```python
from build123d import *

# Parameters (mm, degrees)
SKETCH1_W           = 70
SKETCH1_H           = 75
BOSS_EXTRUDE1_DEPTH = 9
SKETCH2_W           = 65.1
SKETCH2_H           = 70.1
CUT_EXTRUDE1_DEPTH  = 4
SKETCH4_R           = 2.5
BOSS_EXTRUDE3_DEPTH = 7.5
FILLET1_R           = 0.4


with BuildPart() as part:
    # Sketch1 → Boss-Extrude1 (new body)
    with BuildSketch(Plane(origin=(0, 0, 0), x_dir=(1, 0, 0), z_dir=(0, 1, 0))):
        with Locations((35, 37.5)):
            Rectangle(SKETCH1_W, SKETCH1_H)
    extrude(amount=BOSS_EXTRUDE1_DEPTH)

    # Sketch2 → Cut-Extrude1 (cut)
    with BuildSketch(Plane(origin=(0, 9, 0), x_dir=(1, 0, 0), z_dir=(0, 1, 0))):
        with Locations((35, 37.5)):
            Rectangle(SKETCH2_W, SKETCH2_H)
    extrude(amount=-CUT_EXTRUDE1_DEPTH, mode=Mode.SUBTRACT)

    # Sketch4 → Boss-Extrude3 (add)
    with BuildSketch(Plane.XZ):
        with Locations(Location((17.5, -54, 0), (0, 0, 270))):
            Circle(SKETCH4_R)
        with Locations(Location((52.5, -54, 0), (0, 0, 90))):
            Circle(SKETCH4_R)
    extrude(amount=BOSS_EXTRUDE3_DEPTH)

    # Fillet1
    fillet1_edges = [part.edges().sort_by_distance(p)[0] for p in [
        (70, 9, -37.5),
        (35, 9, -75),
        (2.45, 7, -72.55),
        (2.45, 7, -2.45),
        (67.55, 7, -2.45),
        (67.55, 7, -72.55),
        (17.5, 0, -51.5),
        (17.5, -7.5, -51.5),
        (52.5, 0, -56.5),
        (52.5, -7.5, -56.5),
        (0, 9, -37.5),
        (35, 0, -75),
        (70, 0, -37.5),
        (35, 0, 0),
        (0, 0, -37.5),
        (0, 4.5, -75),
        (70, 4.5, -75),
        (70, 4.5, 0),
        (0, 4.5, 0),
        (35, 9, 0),
    ]]
    fillet(fillet1_edges, radius=FILLET1_R)


solid = part.part
```
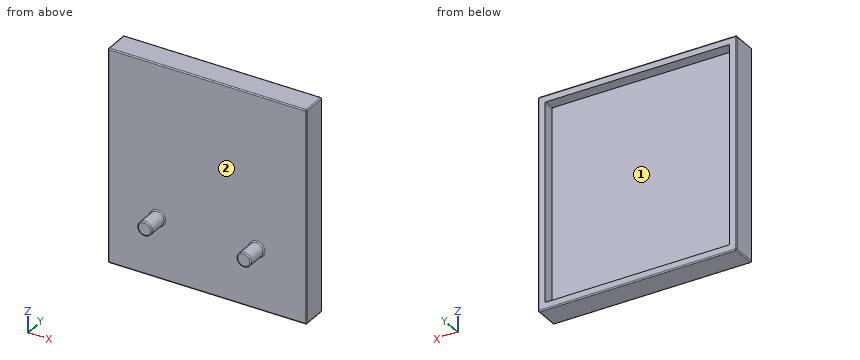
Design review of the part built by this model. Coordinates are the model's own, in mm. Face numbers are marked on the shaded views. Round coordinates to 2 decimals unless told otherwise and drop trailing zeros. Write each loop counter-clockwise with the first axis right and the second up, starting at its lowest first coordinate (ties: lowest second). Pieces come first, ordered by that corner, then holes. Notation, with made-up numbers: (14, 61) -> (32, 61) arc R18 cw to (32, 78) -> close; hole circle Ø4 at (5.25, 62.5). An arc over 180 degrees is marked (long way). Answer in a Markdown table with one row per item.
Q1. To check wall thickness, follow L1, parallel to Z at x = 11, y = 5.5; L2, parallel to X at y = 5.25, z = -28.5; L3, parallel to X at y = -1.5, z = -54. State the ranges of each line that lie inside material, in increasing order. Write a range as [from, to].
The answers:
| item | result |
|---|---|
| L1 | [-75, -72.55], [-2.45, 0] |
| L2 | [0, 2.45], [67.55, 70] |
| L3 | [15, 20], [50, 55] |
Q2. Clearance check with flat-ended pins moving along their axes: pin 1 Ø2 at (x, z) = (59, -22) entering from +Y; pin 2 Ø5 at (x, y) = (60, 7) entering from +Z; pin 3 Ø2 at (x, z) = (39.5, -57.5) entering from -Y. State where each tip first meets the part, or that it passes through.
The answers:
| item | result |
|---|---|
| pin 1 | y = 5 |
| pin 2 | z = 0 |
| pin 3 | y = 0 |
Q3. Take a section at B-B, the plane x = 36. State the section outline as (y, z) points.
The answers:
| item | result |
|---|---|
| outline | (0, -74.6) arc R0.4 ccw to (0.4, -75) -> (8.6, -75) arc R0.4 ccw to (9, -74.6) -> (9, -72.55) -> (5, -72.55) -> (5, -2.45) -> (9, -2.45) -> (9, -0.4) arc R0.4 ccw to (8.6, 0) -> (0.4, 0) arc R0.4 ccw to (0, -0.4) -> close |
Q4. Draft analysis for pull direction Z (two halves, no side actions). For the marked faces 1 and 2, state which applies: +Z half, -Z half, draft (parallel to the pull), parting line (faces both ways), or undercut.
The answers:
| item | result |
|---|---|
| face 1 | undercut |
| face 2 | draft |
Q5. Take a section at C-C, the plane y = -6. State the section outline as (x, z) points.
The answers:
| item | result |
|---|---|
| outline | circle Ø5 at (17.5, -54); circle Ø5 at (52.5, -54) |
Q6. Take a section at A-A, the plane z = -16. State the section outline as (x, y) points, then the cut area to 3 significant figures.
The answers:
| item | result |
|---|---|
| outline | (0, 0.4) arc R0.4 ccw to (0.4, 0) -> (69.6, 0) arc R0.4 ccw to (70, 0.4) -> (70, 8.6) arc R0.4 ccw to (69.6, 9) -> (67.55, 9) -> (67.55, 5) -> (2.45, 5) -> (2.45, 9) -> (0.4, 9) arc R0.4 ccw to (0, 8.6) -> close |
| area | 369 mm² |
Q7. Take a section at D-D, the plane x = 52.5. State the section outline as (y, z) points, then the cut area to 3 significant figures.
The answers:
| item | result |
|---|---|
| outline | (-7.5, -56.1) arc R0.4 ccw to (-7.1, -56.5) -> (-0.4, -56.5) arc R0.4 cw to (0, -56.9) -> (0, -74.6) arc R0.4 ccw to (0.4, -75) -> (8.6, -75) arc R0.4 ccw to (9, -74.6) -> (9, -72.55) -> (5, -72.55) -> (5, -2.45) -> (9, -2.45) -> (9, -0.4) arc R0.4 ccw to (8.6, 0) -> (0.4, 0) arc R0.4 ccw to (0, -0.4) -> (0, -51.1) arc R0.4 cw to (-0.4, -51.5) -> (-7.1, -51.5) arc R0.4 ccw to (-7.5, -51.9) -> close |
| area | 432 mm² |
